The listing builds one solid part. Answer for the finished solid, in the listing's coordinates (mm). A direction names the side the tool comes from. Give positions to 0.01 mm unless a question says otherwise; leave off trailing zeros. Write each loop counter-clockwise with the first axis right and the second up, starting at its lowest first coordinate (ties: lowest second). Pieces come first, ordered by that corner, then holes. Notation, with made-up numbers: (14, 32) - (26, 32) arc R18 cw to (26, 45) - close; hole circle Ø1 at (73.25, -13). An arc over 180 degrees is marked (long way). Answer as CSV lines item,"result". Start each with the question number.
(1) Straight lines are drawn through the part: probe 1 along Z at (x, y) = (-4.5, 0.5); probe 2 along Z at (x, y) = (-5.75, -1); probe 3 along Z at (x, y) = (1, 1.75). For each, find the intervals that lie inside material, in ascending order.
(2) Each of these flat-tipped pins is pushed along its axis until it touches: pin 1 Ø3 at (x, y) = (-1, -1.5) entering from +Z; pin 2 Ø8 at (y, z) = (7, -2.5) entering from +X; pin 3 Ø5 at (y, z) = (8, 4.5) entering from -X. Where does it stop, or does it pass through?
(3) For faces 4 (the face through (0, -4.268, -6)), 5 (the face through (0, -5.042, 6)), 6 (the face through (-4, 2, 7)), 7 (the face through (0, -4.268, 6)), 8 (the face through (-4, -3.07, 4.24)), determine the directions among +Z, -Z, +X, -X, +Y, -Y from which every point of the face is accessible in a straight line to the end or side of a thin tool.
(4) Find section B-B (z = -5.5). Write down the section's boundary in (x, y).
(5) Find section D-D (z = 4.5). Write down the section's boundary in (x, y), then the cut area to 3 significant figures.
(6) Find section C-C (y = -2.5). Write down the section's boundary in (x, z).
(7) Find section A-A (y = 8). Write down the section's boundary in (x, z).
(8) For a pull along X with two mould halves and no side action, classify faces 1 (the face through (-4, 2, -7)), 2 (the face through (-4, -3.07, -4.24)), 3 (the face through (0, 0, -5)) as pulls with the +X half, pulls with the -X half, needs draft (parallel to the pull), parting line crosses it, or undercut.
from build123d import *

# Parameters (mm, degrees)
F0_R     = 4
F1_DEPTH = 3.5
F2_R     = 5.0416218024
F2_R_2   = 4
F3_DEPTH = 1.5
F5_DEPTH = 2


with BuildPart() as f1:
    # F0 (on Top) → F1 (new body)
    with BuildSketch(Plane.XY):
        Circle(F0_R)
    extrude(amount=F1_DEPTH)

    # F2 (on face) → F3 (join)
    with BuildSketch(Plane.XY.offset(3.5)):
        Circle(F2_R)
        Circle(F2_R_2, mode=Mode.SUBTRACT)
        Circle(F2_R_2)
    extrude(amount=F3_DEPTH)

    # F4 (on face) → F5 (join)
    with BuildSketch(Plane.XY.offset(5)):
        with BuildLine():
            ThreePointArc((-2.3542444359, 4.4581928553), (-3.4970506358, 3.6316094571), (-4.3661725175, 2.5208109698))
            ThreePointArc((-4.3661725175, 2.5208109698), (-4.8935913453, 1.2127300373), (-5.0380304856, -0.1902609394))
            Line((-5.0380304856, -0.1902609394), (-2.3542444359, 4.4581928553))
        make_face()
        with BuildLine():
            ThreePointArc((-2.6837860497, -4.2679319158), (-1.3965406905, -4.8443394285), (0, -5.0416218024))
            ThreePointArc((0, -5.0416218024), (1.3965406905, -4.8443394285), (2.6837860497, -4.2679319158))
            Line((2.6837860497, -4.2679319158), (-2.6837860497, -4.2679319158))
        make_face()
        with BuildLine():
            ThreePointArc((5.0416218024, 0), (4.8698327257, 1.3048676647), (4.3661726358, 2.5208107651))
            ThreePointArc((4.3661726358, 2.5208107651), (3.497050721, 3.6316093751), (2.3542444359, 4.4581928553))
            Line((2.3542444359, 4.4581928553), (5.0380304856, -0.1902609394))
            ThreePointArc((5.0380304856, -0.1902609394), (5.0407238932, -0.0951474154), (5.0416218024, 0))
        make_face()
        with BuildLine():
            ThreePointArc((2.3542444359, 4.4581928553), (3.497050721, 3.6316093751), (4.3661726358, 2.5208107651))
            Line((4.3661726358, 2.5208107651), (0, 10.0832436048))
            Line((0, 10.0832436048), (-4.3661725175, 2.5208109698))
            ThreePointArc((-4.3661725175, 2.5208109698), (-3.4970506358, 3.6316094571), (-2.3542444359, 4.4581928553))
            Line((-2.3542444359, 4.4581928553), (0, 8.5358638316))
            Line((0, 8.5358638316), (2.3542444359, 4.4581928553))
        make_face()
        with BuildLine():
            Line((-8.7323451143, -5.0416218024), (0, -5.0416218024))
            ThreePointArc((0, -5.0416218024), (-1.3965406905, -4.8443394285), (-2.6837860497, -4.2679319158))
            Line((-2.6837860497, -4.2679319158), (-7.3922749214, -4.2679319158))
            Line((-7.3922749214, -4.2679319158), (-5.0380304856, -0.1902609394))
            ThreePointArc((-5.0380304856, -0.1902609394), (-4.8935913453, 1.2127300373), (-4.3661725175, 2.5208109698))
            Line((-4.3661725175, 2.5208109698), (-8.7323451143, -5.0416218024))
        make_face()
        with BuildLine():
            Line((0, -5.0416218024), (8.7323451143, -5.0416218024))
            Line((8.7323451143, -5.0416218024), (4.3661726358, 2.5208107651))
            ThreePointArc((4.3661726358, 2.5208107651), (4.8698327257, 1.3048676647), (5.0416218024, 0))
            ThreePointArc((5.0416218024, 0), (5.0407238932, -0.0951474154), (5.0380304856, -0.1902609394))
            Line((5.0380304856, -0.1902609394), (7.3922749214, -4.2679319158))
            Line((7.3922749214, -4.2679319158), (2.6837860497, -4.2679319158))
            ThreePointArc((2.6837860497, -4.2679319158), (1.3965406905, -4.8443394285), (0, -5.0416218024))
        make_face()
    extrude(amount=F5_DEPTH)

    # F6: F1 across plane


with BuildPart() as f1_1:
    add(f1.part)
    add(f1.part.mirror(Plane.XY))


solid = f1_1.part
Result set:
1,probe 1,"-5 to -3.5, 3.5 to 5"
1,probe 2,"-7 to -5, 5 to 7"
1,probe 3,"-5 to 5"
2,pin 1,"z = 5"
2,pin 2,"x = 3.95"
2,pin 3,"x = -2.62"
3,face 4,"-Z"
3,face 5,"+Z, -Z, +X, -X, -Y"
3,face 6,"+Z, +X, -X, +Y, -Y"
3,face 7,"+Z"
3,face 8,"none"
4,outline,"(-8.73, -5.04) - (8.73, -5.04) - (0, 10.08) - close; hole (-7.39, -4.27) - (7.39, -4.27) - (0, 8.54) - close"
5,outline,"circle Ø10.08 at (0, 0)"
5,area,"79.9 mm^2"
6,outline,"(-7.26, -7) - (-6.37, -7) - (-6.37, -5) - (-7.26, -5) - close; (-7.26, 5) - (-6.37, 5) - (-6.37, 7) - (-7.26, 7) - close; (-4.38, -5) - (4.38, -5) - (4.38, -3.5) - (3.12, -3.5) - (3.12, 3.5) - (4.38, 3.5) - (4.38, 5) - (-4.38, 5) - (-4.38, 3.5) - (-3.12, 3.5) - (-3.12, -3.5) - (-4.38, -3.5) - close; (6.37, -7) - (7.26, -7) - (7.26, -5) - (6.37, -5) - close; (6.37, 5) - (7.26, 5) - (7.26, 7) - (6.37, 7) - close"
7,outline,"(-1.2, -7) - (-0.31, -7) - (-0.31, -5) - (-1.2, -5) - close; (-1.2, 5) - (-0.31, 5) - (-0.31, 7) - (-1.2, 7) - close; (0.31, -7) - (1.2, -7) - (1.2, -5) - (0.31, -5) - close; (0.31, 5) - (1.2, 5) - (1.2, 7) - (0.31, 7) - close"
8,face 1,"needs draft"
8,face 2,"parting line crosses it"
8,face 3,"undercut"
